Geometry check sheet. Reference: the model listing, model coordinates, mm. Face numbers are marked on the shaded views. A direction names the side the tool comes from. Round coordinates to 2 decimals unless told otherwise and drop trailing zeros. Loops run counter-clockwise (first coordinate to the right, second up) from the corner with the lowest first, then second, coordinate; pieces in that order, holes last. Notation, with made-up numbers: (-3, 76) -> (30, 76) arc R3 ccw to (30, 80) -> close; hole circle Ø8 at (-9.5, 76.25). An arc over 180 degrees is marked (long way). Use a Markdown table: item, result. Add a question column.
Q1. Material ranges on L1, parallel to X at y = 10.1, z = 0.55; L2, parallel to X at y = -9, z = -7.5; L3, parallel to X at y = -17.85, z = -13.5, recorded low to high.
Q2. Sectioned sample at D-D, the plane y = -3.9. Enter the section's corners in (x, z), then the cut area to 3 significant figures.
Q3. Set-up check for the marked faces 1 and 2: record each of +Z, -Z, +X, -X, +Y, -Y from which the full face is reachable in a straight line by a thin tool's end or side.
Q4. Gauge pin test, flat ends, axial feed: P1, Ø6, axis at x = 9, z = -14, coming from the +Y side; P2, Ø7, axis at x = 9, y = -9.9, coming from the -Z side; P3, Ø1, axis at x = 1, y = -10.5, coming from the -Z side. Record the tip position at first contact, or that the pin passes through.
Q5. Sectioned sample at A-A, the plane y = 10.1. Enter the section's corners in (x, z), then the cut area to 3 significant figures.
Q6. Sectioned sample at C-C, the plane z = -13.5. Enter the section's corners in (x, y), then the cut area to 3 significant figures.
Q7. Sectioned sample at B-B, the plane x = 26. Enter the section's corners in (y, z), then the cut area to 3 significant figures.
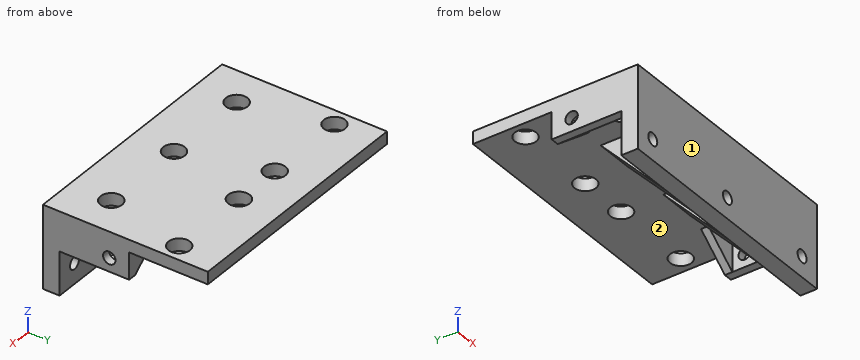
```python
from build123d import *

# Parameters (mm, degrees)
EXTRUDE_1_DEPTH     = 60
SKETCH_2_W          = 15
SKETCH_2_H          = 17
SKETCH_2_W_2        = 12
CUT_EXTRUDE_1_DEPTH = 60
HOLE_WIZARD_1_D     = 5.2
HOLE_WIZARD_2_D     = 3
SKETCH_7_R          = 1.5
EXTRUDE_2_DEPTH     = 2
EXTRUDE_3_DEPTH     = 1.8
HOLE_WIZARD_3_D     = 5.2


with BuildPart() as part:
    # 草图1 → 凸台-拉伸1 (new body)
    with BuildSketch(Plane(origin=(0, 0, 0), x_dir=(0, 0, -1), z_dir=(1, 0, 0))):
        Polygon((-1.5, 19.9), (1.5, 19.9), (1.5, -0.1), (18.5, -15.9), (18.5, -19.9), (1.5, -19.9), (-1.5, -19.9), align=None)
    extrude(amount=EXTRUDE_1_DEPTH)

    # 草图2 → 切除-拉伸1 (cut)
    with BuildSketch(Plane(origin=(0, -15.9, 0), x_dir=(-1, 0, 0), z_dir=(0, -1, 0))):
        with Locations((-52.5, 10)):
            Rectangle(SKETCH_2_W, SKETCH_2_H)
        with Locations((-7.5, 10)):
            Rectangle(SKETCH_2_W, SKETCH_2_H)
        with Locations((-30, 10)):
            Rectangle(SKETCH_2_W_2, SKETCH_2_H)
    extrude(amount=-CUT_EXTRUDE_1_DEPTH, mode=Mode.SUBTRACT)

    # 孔1 (through all)
    with Locations(Plane(origin=(0, 0, -1.5), x_dir=(-1, 0, 0), z_dir=(0, 0, -1))):
        with Locations((-51, -9.9), (-30, -9.9), (-9, -9.9)):
            Hole(HOLE_WIZARD_1_D / 2)

    # 孔2 (through all)
    with Locations(Plane(origin=(0, -19.9, 0), x_dir=(-1, 0, 0), z_dir=(0, -1, 0))):
        with Locations((-55, 13.5), (-30, 13.5), (-5, 13.5)):
            Hole(HOLE_WIZARD_2_D / 2)

    # 草图7 → 凸台-拉伸2 (add)
    with BuildSketch(Plane.ZY):
        Polygon((-1.5, -0.9), (-8, -0.9), (-8, -6.9), (-8, -15.9), (-1.5, -15.9), (-1.5, -6.9), align=None)
        with Locations((-4.75, -3.9)):
            Circle(SKETCH_7_R, mode=Mode.SUBTRACT)
    extrude_2 = extrude(amount=-EXTRUDE_2_DEPTH)

    # 草图8 → 凸台-拉伸3 (add)
    with BuildSketch(Plane(origin=(0, -0.9, 0), x_dir=(1, 0, 0), z_dir=(0, 1, 0))):
        Polygon((2, 8), (10, 1.5), (2, 1.5), (0, 1.5), (0, 8), align=None)
    extrude_3 = extrude(amount=EXTRUDE_3_DEPTH)

    # 孔3 (through all)
    with Locations(Plane(origin=(56, 10.1, -1.5), x_dir=(0, -1, 0), z_dir=(0, 0, -1))):
        with Locations((0, 0), (0, 20), (0, 32), (0, 52)):
            Hole(HOLE_WIZARD_3_D / 2)

    # 镜向1: 凸台-拉伸2, 凸台-拉伸3 across plane
    add(extrude_2.mirror(Plane.ZY.offset(-30)))
    add(extrude_3.mirror(Plane.ZY.offset(-30)))


solid = part.part
```
Values:
| question | item | result |
|---|---|---|
| 1 | L1 | 0 to 1.4, 6.6 to 21.4, 26.6 to 33.4, 38.6 to 53.4, 58.6 to 60 |
| 1 | L2 | 0 to 2, 15 to 24, 36 to 45, 58 to 60 |
| 1 | L3 | 0 to 3.5, 6.5 to 28.5, 31.5 to 53.5, 56.5 to 60 |
| 2 | outline | (0, -8) -> (2, -8) -> (2, -6.25) -> (0, -6.25) -> close; (0, -3.25) -> (2, -3.25) -> (2, -1.5) -> (15, -1.5) -> (15, -5.59) -> (24, -5.59) -> (24, -1.5) -> (36, -1.5) -> (36, -5.59) -> (45, -5.59) -> (45, -1.5) -> (58, -1.5) -> (58, -3.25) -> (60, -3.25) -> (60, 1.5) -> (0, 1.5) -> close; (58, -8) -> (60, -8) -> (60, -6.25) -> (58, -6.25) -> close |
| 2 | area | 268 mm^2 |
| 3 | face 1 | +Z, -Z, +X, -X, -Y |
| 3 | face 2 | -Z |
| 4 | P1 | y = -15.9 |
| 4 | P2 | z = -1.5 |
| 4 | P3 | z = -8 |
| 5 | outline | (0, -1.5) -> (1.4, -1.5) -> (1.4, 1.5) -> (0, 1.5) -> close; (6.6, -1.5) -> (21.4, -1.5) -> (21.4, 1.5) -> (6.6, 1.5) -> close; (26.6, -1.5) -> (33.4, -1.5) -> (33.4, 1.5) -> (26.6, 1.5) -> close; (38.6, -1.5) -> (53.4, -1.5) -> (53.4, 1.5) -> (38.6, 1.5) -> close; (58.6, -1.5) -> (60, -1.5) -> (60, 1.5) -> (58.6, 1.5) -> close |
| 5 | area | 118 mm^2 |
| 6 | outline | (0, -19.9) -> (3.5, -19.9) -> (3.5, -15.9) -> (0, -15.9) -> close; (6.5, -19.9) -> (28.5, -19.9) -> (28.5, -15.9) -> (24, -15.9) -> (24, -11.25) -> (15, -11.25) -> (15, -15.9) -> (6.5, -15.9) -> close; (31.5, -19.9) -> (53.5, -19.9) -> (53.5, -15.9) -> (45, -15.9) -> (45, -11.25) -> (36, -11.25) -> (36, -15.9) -> (31.5, -15.9) -> close; (56.5, -19.9) -> (60, -19.9) -> (60, -15.9) -> (56.5, -15.9) -> close |
| 6 | area | 288 mm^2 |
| 7 | outline | (-19.9, -18.5) -> (-15.9, -18.5) -> (-15.9, -1.5) -> (8.44, -1.5) -> (8.44, 1.5) -> (-19.9, 1.5) -> close; (11.76, -1.5) -> (19.9, -1.5) -> (19.9, 1.5) -> (11.76, 1.5) -> close |
| 7 | area | 177 mm^2 |
